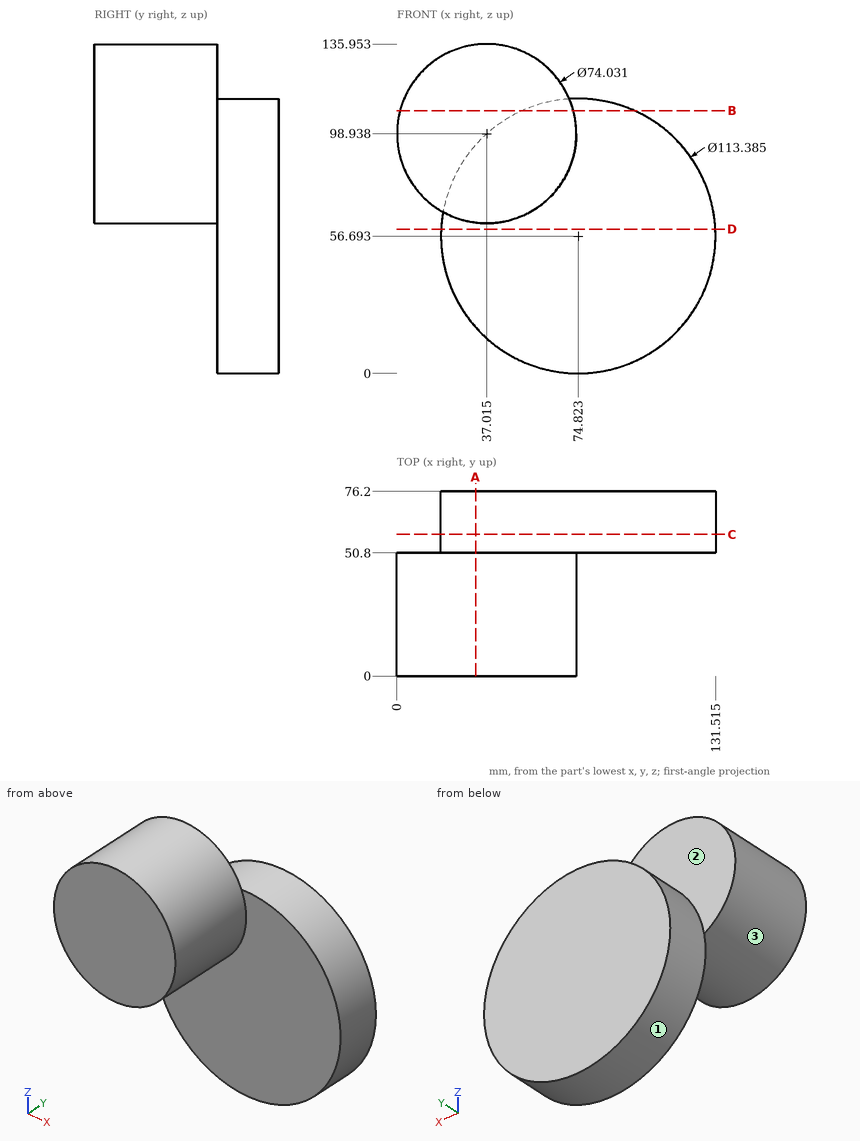
Check sheet for the drawn part. Datum: minimum x, y, z corner. Units: mm. A direction names the side the tool comes from. Give positions to 0.01 mm unless a question says otherwise; leave off trailing zeros. Write each loop counter-clockwise with the first axis right and the second up, starting at its lowest first coordinate (ties: lowest second). Pieces come first, ordered by that corner, then holes. Notation, with made-up numbers: (78.25, -18) -> (97.25, -18) arc R25 cw to (97.25, 18) -> close; hole circle Ø7 at (-20, -6). An arc over 180 degrees is marked (long way). Use one line per item in the form item = value. Start each with the question number.
1. Section check A-A (x = 32.5). Record the cut outline in (y, z), and give its area (3 significant figures).
2. Section check D-D (z = 59.5). Record the cut outline in (x, y) (1 decimal).
3. Thickness scan on line 1 along Y through (x, z) = (74.5, 33.5); line 2 along Y through (x, z) = (32, 98); line 3 along Z through (x, y) = (68, 35) (1 decimal). Record the ranges inside material, lowest first. Write a range as from..to.
4. Go/stop test with flat-tipped pins: P1, Ø1, axis at y = 46, z = 119.5, coming from the -X side; P2, Ø2, axis at x = 35, z = 52.5, coming from the -Y side; P3, Ø10, axis at x = 45.5, y = 18, coming from the +Z side; P4, Ø12, axis at x = 84, y = 31.5, coming from the -Z side. Record where each tip stops, or that it passes through.
5. Section check B-B (z = 108.5). Record the cut outline in (x, y) (1 decimal).
6. Section check C-C (y = 58.5). Record the cut outline in (x, z) (1 decimal), and give its area (3 significant figures).
7. Access from +Z, -Z, +X, -X, +Y, -Y to the whole of each face (thin tool, end or side, straight path). Record for the marked faces 1, 2 and 3.
Conclusion:
q1.outline = (0, 62.2) -> (50.8, 62.2) -> (50.8, 18.97) -> (76.2, 18.97) -> (76.2, 94.41) -> (50.8, 94.41) -> (50.8, 135.68) -> (0, 135.68) -> close
q1.area = 5,650 mm²
q2.outline = (18.2, 50.8) -> (131.4, 50.8) -> (131.4, 76.2) -> (18.2, 76.2) -> close
q3.line_1 = 50.8..76.2
q3.line_2 = 0..50.8
q3.line_3 = 78.7..119.2
q4.P1 = 5.91
q4.P2 = 50.8
q4.P3 = 135.79
q4.P4 = through
q5.outline = (1.3, 0) -> (72.8, 0) -> (72.8, 50.8) -> (97.8, 50.8) -> (97.8, 76.2) -> (51.8, 76.2) -> (51.8, 50.8) -> (1.3, 50.8) -> close
q6.outline = circle Ø113.4 at (74.8, 56.7)
q6.area = 10,100 mm²
q7.face_1 = +Y
q7.face_2 = +Z, -X, +Y
q7.face_3 = -Y
